from build123d import *

# Parameters (mm, degrees)
SKETCH9_W           = 15
SKETCH9_H           = 8.35
BOSS_EXTRUDE4_DEPTH = 80
CUT_EXTRUDE4_DEPTH  = 50
SKETCH10_R          = 2.625
CUT_EXTRUDE5_DEPTH  = 30
SKETCH12_W          = 3
SKETCH12_H          = 3
BOSS_EXTRUDE5_DEPTH = 4.15
SKETCH13_W          = 2
SKETCH13_H          = 3
CUT_EXTRUDE6_DEPTH  = 1
BOSS_EXTRUDE6_DEPTH = 3


with BuildPart() as part:
    # Sketch9 → Boss-Extrude4 (new body)
    with BuildSketch(Plane.XY):
        with Locations((0, 4.175)):
            Rectangle(SKETCH9_W, SKETCH9_H)
    extrude(amount=BOSS_EXTRUDE4_DEPTH)

    # Sketch7 → Cut-Extrude4 (cut)
    with BuildSketch(Plane.XY):
        Polygon((-5.5, 2), (-5.5, 5.35), (-2.5, 5.35), (-2.5, 8.35), (2.5, 8.35), (2.5, 5.35), (5.5, 5.35), (5.5, 2), align=None)
    extrude(amount=CUT_EXTRUDE4_DEPTH, mode=Mode.SUBTRACT)

    # Sketch10 → Cut-Extrude5 (cut)
    with BuildSketch(Plane.XY.offset(80)):
        with Locations((0, 4.625)):
            Circle(SKETCH10_R)
    extrude(amount=-CUT_EXTRUDE5_DEPTH, mode=Mode.SUBTRACT)

    # Sketch12 → Boss-Extrude5 (add)
    with BuildSketch(Plane(origin=(7.5, 0, 0), x_dir=(0, 0, -1), z_dir=(1, 0, 0))):
        with Locations((-75.5, 3.64)):
            Rectangle(SKETCH12_W, SKETCH12_H)
    boss_extrude5 = extrude(amount=BOSS_EXTRUDE5_DEPTH)

    # Sketch13 → Cut-Extrude6 (cut)
    with BuildSketch(Plane.XY.offset(77)):
        with Locations((9.575, 3.64)):
            Rectangle(SKETCH13_W, SKETCH13_H)
    cut_extrude6 = extrude(amount=-CUT_EXTRUDE6_DEPTH, mode=Mode.SUBTRACT)

    # Mirror2: Boss-Extrude5 across plane
    add(boss_extrude5.mirror(Plane(origin=(0, 0, 0), x_dir=(0, 0, 1), z_dir=(1, 0, 0))))

    # Mirror4: Cut-Extrude6 across plane
    add(cut_extrude6.mirror(Plane(origin=(0, 0, 0), x_dir=(0, 0, 1), z_dir=(1, 0, 0))), mode=Mode.SUBTRACT)

    # Sketch14 → Boss-Extrude6 (add)
    with BuildSketch(Plane(origin=(0, 5.14, 0), x_dir=(1, 0, 0), z_dir=(0, 1, 0))):
        Polygon((11.65, -74), (7.5, -69.685450349), (7.5, -74), align=None)
    boss_extrude6 = extrude(amount=-BOSS_EXTRUDE6_DEPTH)

    # Mirror5: Boss-Extrude6 across plane
    add(boss_extrude6.mirror(Plane(origin=(0, 0, 0), x_dir=(0, 0, 1), z_dir=(1, 0, 0))))


solid = part.part
Geometry: final body of the model. Coordinates: model frame, mm. A direction names the side the tool comes from. Round coordinates to 2 decimals unless told otherwise and drop trailing zeros. Loops run counter-clockwise (first coordinate to the right, second up) from the corner with the lowest first, then second, coordinate; pieces in that order, holes last. Notation, with made-up numbers: (85.25, 71) - (94.25, 71) arc R33 ccw to (94.25, 109) - close; hole circle Ø7 at (31, 63.25). An arc over 180 degrees is marked (long way). Write each question's results on one line, items separated by ' | '. Start each with the question number.
1) Cut plane C-C on x = -4. Return loops of the section in (y, z), then the cut area to 4 significant figures.
2) Cut plane A-A on y = 6.5. Return loops of the section in (x, z).
3) Cut plane D-D on z = 67. Return loops of the section in (x, y) (3 decimals), then the cut area to 3 significant figures.
4) Cut plane B-B on z = 42.5. Return loops of the section in (x, y).
5) First-contact query: P1, Ø3.5, axis at x = -9.5, z = 74.5, coming from the +Y side; P2, Ø2, axis at x = -9.5, z = 75, coming from the -Y side; P3, Ø3.5, axis at y = 7, z = 15, coming from the -X side. Flat tips, straight axial feed; report the tip coordinate or a pass-through.
6) Line query: probe 1 along X at (y, z) = (6, 15.5); probe 2 along X at (y, z) = (4.5, 10.5); probe 3 along Y at (x, z) = (0, 60). Output: solid intervals per line, ascending. Write a range as [from, to].
7) Mould query, pull axis X, two halves, no side actions, for faces 5 (the face through (11.65, 4, 76)), 6 (the face through (10, 4, 76)), 7 (the face through (0, 1, 0)), 8 (the face through (-11.65, 4, 76)). Classes: released by +X, released by -X, zero draft, split by the parting line, or undercut.
8) Access query for faces 1 (the face through (-4, 4, 50)), 2 (the face through (9, 2.14, 74)), 3 (the face through (2.5, 7, 25)), 4 (the face through (-10, 4, 76)). Directions: +Z, -Z, +X, -X, +Y, -Y. A direction counts if a zero-diameter tool reaches every point of the face in a straight line with its end or side. Return the directions, or none.
Verdict:
1) outline: (0, 0) - (2, 0) - (2, 50) - (5.35, 50) - (5.35, 0) - (8.35, 0) - (8.35, 80) - (0, 80) - close | area: 500.5 mm2
2) outline: (-7.5, 0) - (-2.5, 0) - (-2.5, 50) - (-1.84, 50) - (-1.84, 80) - (-7.5, 80) - close; (1.84, 50) - (2.5, 50) - (2.5, 0) - (7.5, 0) - (7.5, 80) - (1.84, 80) - close
3) outline: (-7.5, 0) - (7.5, 0) - (7.5, 8.35) - (-7.5, 8.35) - close; hole circle Ø5.25 at (0, 4.625) | area: 104 mm2
4) outline: (-7.5, 0) - (7.5, 0) - (7.5, 8.35) - (2.5, 8.35) - (2.5, 5.35) - (5.5, 5.35) - (5.5, 2) - (-5.5, 2) - (-5.5, 5.35) - (-2.5, 5.35) - (-2.5, 8.35) - (-7.5, 8.35) - close
5) P1: stops at y = 5.14 | P2: stops at y = 2.14 | P3: stops at x = -7.5
6) probe 1: x = [-7.5, -2.5], [2.5, 7.5] | probe 2: x = [-7.5, -5.5], [5.5, 7.5] | probe 3: y = [0, 2], [7.25, 8.35]
7) face 5: released by +X | face 6: undercut | face 7: zero draft | face 8: released by -X
8) face 1: -Z | face 2: +Z, -Z, +X, -Y | face 3: -Z, +Y | face 4: +Z, +Y, -Y
